from build123d import *

# Parameters (mm, degrees)
SKETCH1_R              = 5
SKETCH1_R_2            = 3
BOSS_EXTRUDE1_DEPTH    = 50
CUT_EXTRUDE1_START     = 16.3
CUT_EXTRUDE1_OUTLINE_R = 3
CUT_EXTRUDE1_DEPTH     = 17.4
SKETCH2_W              = 5.2
SKETCH2_H              = 5
CUT_EXTRUDE2_DEPTH     = 17.4
CUT_EXTRUDE4_DEPTH     = 17.4
SKETCH3_R              = 4.25
BOSS_EXTRUDE2_DEPTH    = 11
SKETCH6_R              = 4.25
CUT_EXTRUDE5_DEPTH     = 59.883359407
HOLE1_D                = 4.8
HOLE1_CSINK_D          = 7.75
HOLE1_CSINK_ANGLE      = 82
SKETCH9_R              = 3
BOSS_EXTRUDE3_DEPTH    = 16.3
MIRROR1_START          = 33.7
MIRROR1_OUTLINE_R      = 3
MIRROR1_DEPTH          = 16.3
HOLE2_D                = 4
HOLE2_DEPTH            = 16.3
HOLE2_CSINK_D          = 7.75
HOLE2_CSINK_ANGLE      = 82
HOLE3_D                = 3.8


# Read off the part's stored shape, not the designer's step: Cut-Extrude1, Mirror1
with BuildPart() as part:
    # Sketch1 → Boss-Extrude1 (new body)
    # profile 1 of 2: a face of its own
    with BuildSketch(Plane.XY):
        with BuildLine():
            Line((-2.5, 14.790199458), (-2.5, 24.874685928))
            ThreePointArc((-2.5, 24.874685928), (-24.968651828, -1.251569376), (0, -25))
            ThreePointArc((0, -25), (-5, -20), (0, -15))
            ThreePointArc((0, -15), (-14.947457842, -1.254393904), (-2.5, 14.790199458))
        make_face()
    # profile 2 of 2: a face of its own
    with BuildSketch(Plane.XY):
        with Locations((0, -20)):
            Circle(SKETCH1_R)
        with Locations((0, -20)):
            Circle(SKETCH1_R_2, mode=Mode.SUBTRACT)
    extrude(amount=BOSS_EXTRUDE1_DEPTH)

    # Cut-Extrude1 outline → Cut-Extrude1 (cut)
    with BuildSketch(Plane.XY.offset(CUT_EXTRUDE1_START)):
        with BuildLine():
            ThreePointArc((-1.235879849, -14.949), (-5.196630355, -19.812829077), (-1.59605733, -24.949))
            ThreePointArc((-1.59605733, -24.949), (-0.798435971, -24.987246747), (0, -25))
            ThreePointArc((0, -25), (5, -20), (0, -15))
            ThreePointArc((0, -15), (-0.618465844, -14.987244577), (-1.235879849, -14.949))
        make_face()
        with Locations((0, -20)):
            Circle(CUT_EXTRUDE1_OUTLINE_R, mode=Mode.SUBTRACT)
    extrude(amount=CUT_EXTRUDE1_DEPTH, mode=Mode.SUBTRACT)

    # Sketch2 → Cut-Extrude2 (cut)
    with BuildSketch(Plane.XY.offset(16.3)):
        with Locations((-2.6, -22.5)):
            Rectangle(SKETCH2_W, SKETCH2_H)
    extrude(amount=CUT_EXTRUDE2_DEPTH, mode=Mode.SUBTRACT)

    # Sketch4 → Cut-Extrude4 (cut)
    with BuildSketch(Plane(origin=(0, 0, 33.7), x_dir=(-1, 0, 0), z_dir=(0, 0, -1))):
        with BuildLine():
            Line((2.655027114, -15.763157895), (2.655027114, -14.763157895))
            ThreePointArc((2.655027114, -14.763157895), (1.332784975, -14.940672147), (0, -15))
            ThreePointArc((0, -15), (1.381265629, -15.194575434), (2.655027114, -15.763157895))
        make_face()
    extrude(amount=CUT_EXTRUDE4_DEPTH, mode=Mode.SUBTRACT)

    # Sketch3 → Boss-Extrude2 (add)
    with BuildSketch(Plane(origin=(-2.5, 0, 0), x_dir=(0, 0, -1), z_dir=(1, 0, 0))):
        with Locations((-37.5, 19.832442693)):
            Circle(SKETCH3_R)
    extrude(amount=-BOSS_EXTRUDE2_DEPTH)

    # Sketch6 → Cut-Extrude5 (cut, through all)
    with BuildSketch(Plane.ZY.offset(13.5)):
        with Locations((37.5, 19.832442693)):
            Circle(SKETCH6_R)
    extrude(amount=CUT_EXTRUDE5_DEPTH, mode=Mode.SUBTRACT)

    # Hole1 (through all)
    with Locations(Plane(origin=(-13.5, 19.832442693, 37.5), x_dir=(0, 0, -1), z_dir=(-1, 0, 0))):
        with Locations((0, 0)):
            CounterSinkHole(HOLE1_D / 2, HOLE1_CSINK_D / 2, counter_sink_angle=HOLE1_CSINK_ANGLE)

    # Sketch9 → Boss-Extrude3 (add)
    with BuildSketch(Plane(origin=(0, 0, 0), x_dir=(-1, 0, 0), z_dir=(0, 0, -1))):
        with Locations(Location((0, -20, 0), (0, 0, 180))):
            Circle(SKETCH9_R)
    extrude(amount=-BOSS_EXTRUDE3_DEPTH)

    # Mirror1 outline → Mirror1 (add)
    with BuildSketch(Plane.XY.offset(MIRROR1_START)):
        with Locations((0, -20)):
            Circle(MIRROR1_OUTLINE_R)
    extrude(amount=MIRROR1_DEPTH)

    # Mirror1 2 outline → Mirror1 2 (revolve)
    with BuildSketch(Plane(origin=(0, 19.832442693, 12.5), x_dir=(0, 1, 0), z_dir=(0, 0, -1))):
        Polygon((2.4, -11.803206599), (3.875, -13.5), (4.25, -13.5), (4.25, -6.708985665), (2.4, -6.708985665), align=None)
    revolve(axis=Axis((0, 19.832442693, 12.5), (1, 0, 0)))

    # Mirror1 3 outline → Mirror1 3 (revolve, cut)
    with BuildSketch(Plane(origin=(0, 19.832442693, 12.5), x_dir=(0, 1, 0), z_dir=(0, 0, -1))):
        Polygon((4.25, -13.5), (3.875, -13.5), (2.4, -11.803206599), (2.4, -2.5), (0, -2.5), (0, -19.550181267), (4.25, -19.550181267), align=None)
    revolve(axis=Axis((0, 19.832442693, 12.5), (1, 0, 0)), mode=Mode.SUBTRACT)

    # Hole2
    with Locations(Plane(origin=(0, -20, 0), x_dir=(-1, 0, 0), z_dir=(0, 0, -1))):
        with Locations((0, 0)):
            CounterSinkHole(HOLE2_D / 2, HOLE2_CSINK_D / 2, depth=HOLE2_DEPTH, counter_sink_angle=HOLE2_CSINK_ANGLE)

    # Hole3 (through all)
    with Locations(Plane(origin=(0, -20, 33.7), x_dir=(-1, 0, 0), z_dir=(0, 0, -1))):
        with Locations((0, 0)):
            Hole(HOLE3_D / 2)


solid = part.part
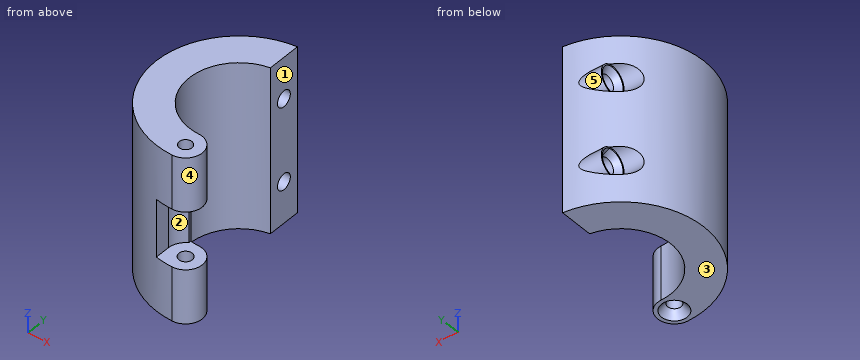
For this review, take the finished solid that the model builds, in its own axes (mm). Face numbers are marked on the shaded views. A direction names the side the tool comes from. Round coordinates to 2 decimals unless told otherwise and drop trailing zeros. Write each loop counter-clockwise with the first axis right and the second up, starting at its lowest first coordinate (ties: lowest second). Pieces come first, ordered by that corner, then holes. Notation, with made-up numbers: (61, 35.5) - (93, 35.5) arc R24 cw to (93, 64.5) - close; hole circle Ø10 at (70, -2.75). An arc over 180 degrees is marked (long way). Use a Markdown table: item, result.
Q1. We need section D-D (z = 4.5). Give the boundary of the cut face in (x, y).
Derived:
| item | result |
|---|---|
| outline | (-2.5, 14.79) - (-2.5, 24.87) arc R25 ccw to (0, -25) arc R5 ccw to (0, -15) arc R15 cw to start; hole circle Ø4 at (0, -20) |
Q2. Machinability: for the marked faces 1, 2, 3, 4 and 5, which of the approach directions +Z, -Z, +X, -X, +Y, -Y give a long, thin tool a straight path to every point of the face, cutting with its end or side? Answer none if there is none.
Derived:
| item | result |
|---|---|
| face 1 | +Z, -Z, +X, +Y |
| face 2 | +X, -Y |
| face 3 | -Z, +X, -X, +Y, -Y |
| face 4 | +Z, -Z, +X |
| face 5 | -X, +Y |
Q3. We need section A-A (z = 37.5). Give the boundary of the cut face in (x, y).
Derived:
| item | result |
|---|---|
| outline | (-19.55, 15.58) arc R25 ccw to (0, -25) arc R5 ccw to (0, -15) arc R15 cw to (-2.5, 14.79) - (-2.5, 17.43) - (-11.8, 17.43) - (-13.5, 15.96) - (-13.5, 15.58) - close; (-13.5, 23.71) - (-11.8, 22.23) - (-2.5, 22.23) - (-2.5, 24.87) arc R25 ccw to (-6.71, 24.08) - (-13.5, 24.08) - close; hole circle Ø3.8 at (0, -20) |
Q4. Clearance check with flat-ended pins moving along their axes: pin 1 (7.5 mm diameter, centred on y = 19.83, z = 12.5, fed in from -X); pin 2 (3 mm diameter, centred on y = -6.5, z = 32.5, fed in from +X); pin 3 (5 mm diameter, centred on x = 0, y = -20, fed in from -Z). State where each tip first meets the part, or that it passes through.
Derived:
| item | result |
|---|---|
| pin 1 | stops at x = -13.36 |
| pin 2 | stops at x = -12.69 |
| pin 3 | stops at z = 1.58 |
Q5. We need section B-B (x = -8). Give the boundary of the cut face in (y, z), plus the area to 3 significant figures.
Derived:
| item | result |
|---|---|
| outline | (-23.69, 0) - (-12.69, 0) - (-12.69, 50) - (-23.69, 50) - close; (12.69, 0) - (23.69, 0) - (23.69, 10.71) arc R4.25 ccw to (23.69, 14.29) - (23.69, 35.71) arc R4.25 ccw to (23.69, 39.29) - (23.69, 50) - (12.69, 50) - close; hole circle Ø4.8 at (19.83, 12.5); hole circle Ø4.8 at (19.83, 37.5) |
| area | 1,070 mm2 |
Q6. Wall thickness on line 1 along X through (y, z) = (-20, 5.5); line 2 along Y through (x, z) = (-10, 11); line 3 along Y through (x, z) = (-5, 37): over which ranges is each line inside the solid? List them lowest first.
Derived:
| item | result |
|---|---|
| line 1 | x = -15 to -2, 2 to 5 |
| line 2 | y = -22.91 to -11.18, 11.18 to 17.96, 21.71 to 23.81 |
| line 3 | y = -24.49 to -14.14, 14.14 to 17.49, 22.18 to 24.49 |
Q7. We need section C-C (z = 12.5). Give the boundary of the cut face in (x, y), plus the area to 3 significant figures.
Derived:
| item | result |
|---|---|
| outline | (-19.55, 15.58) arc R25 ccw to (0, -25) arc R5 ccw to (0, -15) arc R15 cw to (-2.5, 14.79) - (-2.5, 17.43) - (-11.8, 17.43) - (-13.5, 15.96) - (-13.5, 15.58) - close; (-13.5, 23.71) - (-11.8, 22.23) - (-2.5, 22.23) - (-2.5, 24.87) arc R25 ccw to (-6.71, 24.08) - (-13.5, 24.08) - close; hole circle Ø4 at (0, -20) |
| area | 565 mm2 |
